Here's the drawing with two shaded views (mm, measured from the low corner). I have some questions. A direction names the side the tool comes from. Coordinates: 2 decimals unless noted, no trailing zeros. Loops run counter-clockwise (first coordinate to the right, second up) from the corner with the lowest first, then second, coordinate; pieces in that order, holes last. Notation, with made-up numbers: (-5.75, 35) -> (4.25, 35) arc R27 ccw to (4.25, 60) -> close; hole circle Ø10 at (51, 57). An arc over 180 degrees is marked (long way). Answer as a JSON object with one key per item and string values. Group by question number.
Q1. I want a section at A-A on z = 8.5. Write out the boundary of the cut face in (x, y) (1 decimal).
Q2. Thinking about a two-plate mould opening in Y: for the marked faces 1, 2 and 3, which applies, released by +Y, released by -Y, zero draft, split by the parting line, or undercut?
Q3. I'm going to push a flat-ended pin straight in: pin 1 (2 mm diameter, centred on y = 1, z = 5, fed in from +X) (1 decimal). Where does the tip first touch, or does it pass through?
Q4. I want a section at D-D on z = 4. Write out the boundary of the cut face in (x, y).
Q5. I want a section at B-B on x = 7.5. Write out the boundary of the cut face in (y, z) (1 decimal).
Q6. I need wall thicknesses on line 1 (Z direction, x = 11.25, y = 4.5) (1 decimal); line 2 (Z direction, x = 7.5, y = 3.7) (1 decimal); line 3 (X direction, y = 2, z = 8). Which ranges of each line are inside material? Lowest first, please.
Q7. On a 3-axis mill with a long thin cutter (end or side, diameter ignored), from which of +Z, -Z, +X, -X, +Y, -Y can I reach the whole of each face in a straight line? I mean the marked faces 4 and 5. Say none if no direction works.
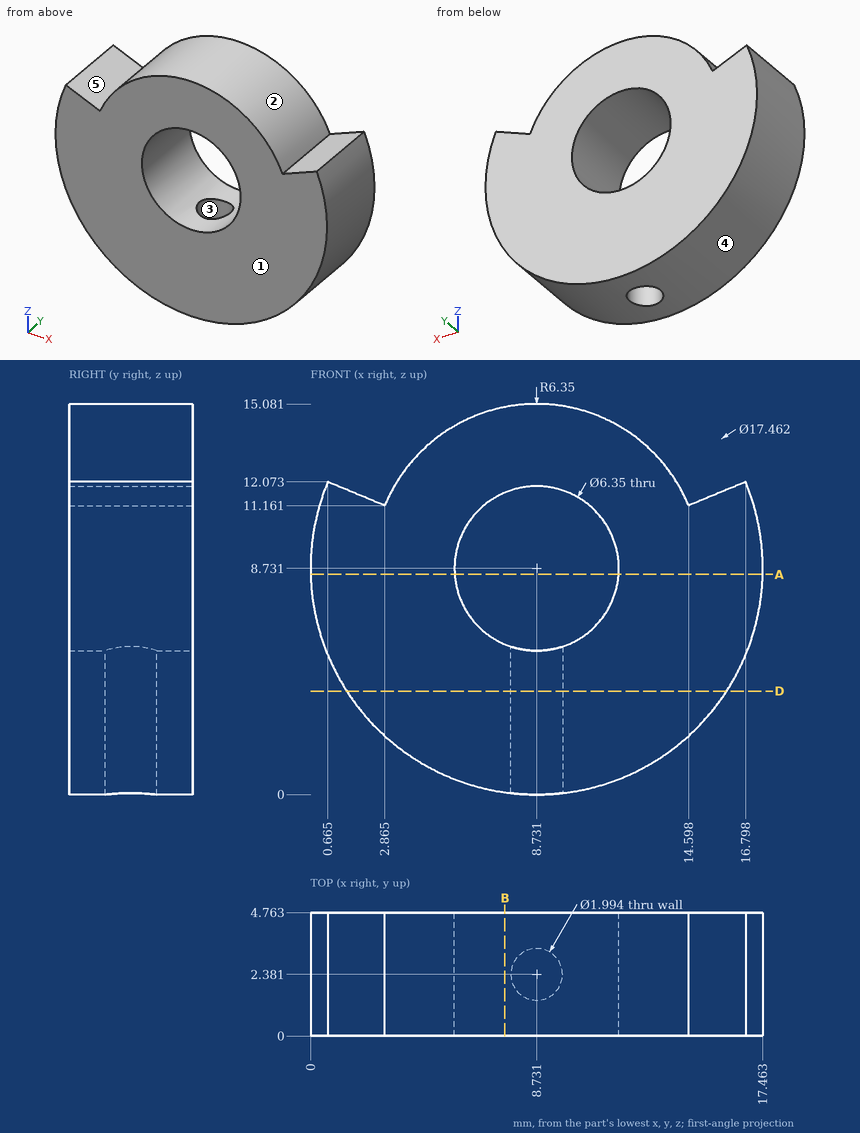
Result set:
{
 "1": {"outline": "(0, 0) -> (5.6, 0) -> (5.6, 4.8) -> (0, 4.8) -> close; (11.9, 0) -> (17.5, 0) -> (17.5, 4.8) -> (11.9, 4.8) -> close"},
 "2": {"face 1": "released by -Y", "face 2": "zero draft", "face 3": "undercut"},
 "3": {"pin 1": "stops at x = 17"},
 "4": {"outline": "(1.39, 0) -> (16.07, 0) -> (16.07, 4.76) -> (1.39, 4.76) -> close; hole circle Ø1.99 at (8.73, 2.38)"},
 "5": {"outline": "(0, 0.1) -> (4.8, 0.1) -> (4.8, 5.8) -> (0, 5.8) -> close; (0, 11.7) -> (4.8, 11.7) -> (4.8, 15) -> (0, 15) -> close"},
 "6": {"line 1": "z = 0.4 to 6.8, 10.7 to 14.6", "line 2": "z = 0.1 to 5.8, 11.7 to 15", "line 3": "x = 0.03 to 5.64, 11.82 to 17.43"},
 "7": {"face 4": "+Y, -Y", "face 5": "+Z, +Y, -Y"}
}
